Can you work these out from the model? Positions are in its coordinate system, mm. Give positions to 0.01 mm unless a question says otherwise; leave off trailing zeros. Order: outer loops, then holes, each group sorted by start corner. A loop starts at its lowest first (then second) coordinate and runs counter-clockwise, first axis right, second up. Notation, with made-up numbers: M 14,9.25 L 44,9.25 A11 ccw 44,29.25 Z; hole C 65,-17.75 d10. An arc over 180 degrees is marked long. One line per question, with ' | ' between items. Start each with the question number.
1) If we section it at C-C, the plane y = -7: Please give me the cut outline in (x, z).
2) I'm going to push flat-ended pins straight in: pin 1 Ø5 at (x, y) = (-7.5, -8) entering from -Z; pin 2 Ø3 at (y, z) = (-2.5, 8.5) entering from -X; pin 3 Ø5 at (x, y) = (0, -6) entering from -Z. Where does each tip first touch, or does it pass through?
3) If we section it at A-A, the plane x = 0: Please give me the cut outline in (y, z), plus the area to 3 significant figures.
4) If we section it at B-B, the plane z = 0: Please give me the cut outline in (x, y), plus the area to 3 significant figures.
5) Thinking about a two-plate mould opening in Z: for faces 1 (the cylindrical face through (-5.78, -4.43, -7.54)), 2 (the cylindrical face through (3.2, -5.3, 10)), 3 (the flat face through (10, 1, -4)), which applies, +Z half, -Z half, draft (parallel to the pull), parting line (faces both ways), or undercut?
6) Please list where these lines run through material, in increasing order: line 1 along X through (y, z) = (-6.25, 0); line 2 along Y through (x, z) = (2, -11); line 3 along Z through (x, y) = (-8, -6.25). Write a range as [from, to].
```python
from build123d import *

# Parameters (mm, degrees)
SKETCH1_R           = 10.5
SKETCH1_R_2         = 9.5
BOSS_EXTRUDE1_DEPTH = 10
BOSS_EXTRUDE2_START = 1
SKETCH2_R           = 12.5
SKETCH2_R_2         = 9.5
BOSS_EXTRUDE2_DEPTH = 1
FILLET1_R           = 0.75


with BuildPart() as part:
    # Sketch1 → Boss-Extrude1 (new body)
    with BuildSketch(Plane(origin=(0, 0, 0), x_dir=(1, 0, 0), z_dir=(0, 1, 0))):
        with Locations(Location((0, 0, 0), (0, 0, 270))):
            Circle(SKETCH1_R)
        with Locations(Location((0, 0, 0), (0, 0, 270))):
            Circle(SKETCH1_R_2, mode=Mode.SUBTRACT)
    extrude(amount=-BOSS_EXTRUDE1_DEPTH)

    # Sketch2 → Boss-Extrude2 (add)
    with BuildSketch(Plane(origin=(0, 0, 0), x_dir=(1, 0, 0), z_dir=(0, 1, 0)).offset(BOSS_EXTRUDE2_START)):
        with Locations(Location((0, 0, 0), (0, 0, 270))):
            Circle(SKETCH2_R)
        with Locations(Location((0, 0, 0), (0, 0, 270))):
            Circle(SKETCH2_R_2, mode=Mode.SUBTRACT)
    extrude(amount=-BOSS_EXTRUDE2_DEPTH)

    # Fillet1
    fillet1_edges = [part.edges().sort_by_distance(p)[0] for p in [
        (0, 1, -12.5),
        (0, 1, -9.5),
        (0, 0, -10.5),
        (0, -10, -9.5),
    ]]
    fillet(fillet1_edges, radius=FILLET1_R)


solid = part.part
```
Results found:
1) outline: C 0,0 d21; hole C 0,0 d19
2) pin 1: stops at z = -9.23 | pin 2: stops at x = -7.83 | pin 3: stops at z = -10.5
3) outline: M -10,-10.5 L -0.75,-10.5 A0.75 cw 0,-11.25 L 0,-12.5 L 0.25,-12.5 A0.75 ccw 1,-11.75 L 1,-10.25 A0.75 ccw 0.25,-9.5 L -9.25,-9.5 A0.75 ccw -10,-10.25 Z; M -10,10.25 A0.75 ccw -9.25,9.5 L 0.25,9.5 A0.75 ccw 1,10.25 L 1,11.75 A0.75 ccw 0.25,12.5 L 0,12.5 L 0,11.25 A0.75 cw -0.75,10.5 L -10,10.5 Z | area: 25.5 mm²
4) outline: M -12.5,0 L -11.25,0 A0.75 cw -10.5,-0.75 L -10.5,-10 L -10.25,-10 A0.75 ccw -9.5,-9.25 L -9.5,0.25 A0.75 ccw -10.25,1 L -11.75,1 A0.75 ccw -12.5,0.25 Z; M 9.5,-9.25 A0.75 ccw 10.25,-10 L 10.5,-10 L 10.5,-0.75 A0.75 cw 11.25,0 L 12.5,0 L 12.5,0.25 A0.75 ccw 11.75,1 L 10.25,1 A0.75 ccw 9.5,0.25 Z | area: 25.5 mm²
5) face 1: undercut | face 2: parting line | face 3: draft
6) line 1: x = [-10.5, -9.5], [9.5, 10.5] | line 2: y = [0, 1] | line 3: z = [-6.8, -5.12], [5.12, 6.8]
